Verification items for the finished model (mm, model axes). A direction names the side the tool comes from. Round coordinates to 2 decimals unless told otherwise and drop trailing zeros. Write each loop counter-clockwise with the first axis right and the second up, starting at its lowest first coordinate (ties: lowest second). Pieces come first, ordered by that corner, then holes. Notation, with made-up numbers: M 28,23 L 42,23 A28 ccw 42,57 Z; hole C -16,-30.5 d9. An arc over 180 degrees is marked long. Answer in a Markdown table with one row per item. Add a question column.
1. Sectioned sample at B-B on y = 2.5. Record the cut outline in (x, z).
2. Set-up check for faces 1 (the flat face through (5.45, -1.7, -2.6)), 2 (the flat face through (4.65, -1.7, -2.6)), 3 (the flat face through (5, 14.1, 0)), 4 (the flat face through (2, 11.6, 0.1)), 5 (the flat face through (9.114, 1.674, 2.454)): record each of +Z, -Z, +X, -X, +Y, -Y from which the full face is reachable in a straight line by a thin tool's end or side.
3. Draft check along Y on faces 6 (the flat face through (9.114, 4.826, -2.546)), 7 (the flat face through (5, -2, -2.034)), 8 (the flat face through (5, 13.9, 8)). Enter one of: pulls with the +Y half, pulls with the -Y half, needs draft (parallel to the pull), parting line crosses it, or undercut.
4. Material ranges on probe 1 along Y at (x, z) = (3, -5.75); probe 2 along Y at (x, z) = (5.25, 2); probe 3 along X at (y, z) = (14, 7.44), recorded low to high.
5. Go/stop test with flat-tipped pins: pin 1 Ø5 at (x, z) = (4, -4) entering from -Y; pin 2 Ø1.2 at (x, z) = (5.5, -1.5) entering from +Y; pin 3 Ø1 at (y, z) = (2.5, -2.5) entering from +X. Record where each tip stops, or that it passes through.
6. Sectioned sample at A-A on z = 2.44. Record the cut outline in (x, y).
7. Sectioned sample at D-D on y = 7.25. Record the cut outline in (x, z), plus the area to 3 significant figures.
8. Sectioned sample at C-C on z = -0.25. Record the cut outline in (x, y).
```python
from build123d import *

# Parameters (mm, degrees)
BOSS_EXTRUDE1_DEPTH          = 10.16
FILLET1_R                    = 0.5
CUT_EXTRUDE1_DEPTH           = 21.100885553
CUT_EXTRUDE1_DEPTH_BACK      = 0.2
SKETCH2_R                    = 1.75
SKETCH3_W                    = 0.8
SKETCH3_H                    = 1.05200998
BOSS_EXTRUDE2_DEPTH          = 3.5
SKETCH4_W                    = 2
SKETCH4_H                    = 3.5
CUT_EXTRUDE2_DEPTH           = 2
CUT_EXTRUDE2_DRAFT           = -10
CUT_EXTRUDE2_PROFILE_2_DEPTH = 2
CUT_EXTRUDE2_PROFILE_2_DRAFT = -10
CUT_EXTRUDE2_PROFILE_3_DEPTH = 2
CUT_EXTRUDE2_PROFILE_3_DRAFT = -10
CUT_EXTRUDE2_PROFILE_4_DEPTH = 2
CUT_EXTRUDE2_PROFILE_4_DRAFT = -10
SKETCH5_W                    = 4.000724796
SKETCH5_H                    = 0.5
CUT_EXTRUDE3_DEPTH           = 0.1


with BuildPart() as part:
    # Sketch1 → Boss-Extrude1 (new, symmetric)
    with BuildSketch(Plane.XY):
        Polygon((0, 9.1), (1.5, 9.1), (2.5, 14.1), (8, 14.1), (9.4, 7), (10.1, 7), (10.1, 0), (0, 0), align=None)
    extrude(amount=BOSS_EXTRUDE1_DEPTH, both=True)

    # Fillet1
    fillet1_edges = [part.edges().sort_by_distance(p)[0] for p in [
        (10.1, 7, 0),
    ]]
    fillet(fillet1_edges, radius=FILLET1_R)

    # Sketch2 → Cut-Extrude1 (cut, two sides: drawn at the far end of the back side and taken through both)
    with BuildSketch(Plane(origin=(0, 14.1, 0), x_dir=(1, 0, 0), z_dir=(0, 1, 0)).offset(-CUT_EXTRUDE1_DEPTH_BACK)):
        with Locations(Location((5.25, 7.56, 0), (0, 0, 90))):
            Circle(SKETCH2_R)
        with Locations(Location((5.25, 2.56, 0), (0, 0, 90))):
            Circle(SKETCH2_R)
        with Locations(Location((5.25, -2.44, 0), (0, 0, 90))):
            Circle(SKETCH2_R)
        with Locations(Location((5.25, -7.44, 0), (0, 0, 90))):
            Circle(SKETCH2_R)
    extrude(amount=CUT_EXTRUDE1_DEPTH + CUT_EXTRUDE1_DEPTH_BACK, mode=Mode.SUBTRACT)

    # Sketch3 → Boss-Extrude2 (add)
    with BuildSketch(Plane.XZ):
        with Locations((5.05, 7.44)):
            Rectangle(SKETCH3_W, SKETCH3_H)
        with Locations((5.05, 2.44)):
            Rectangle(SKETCH3_W, SKETCH3_H)
        with Locations((5.05, -2.56)):
            Rectangle(SKETCH3_W, SKETCH3_H)
        with Locations((5.05, -7.56)):
            Rectangle(SKETCH3_W, SKETCH3_H)
    extrude(amount=BOSS_EXTRUDE2_DEPTH)


with BuildPart() as cut_extrude2_tool:
    # Sketch4 → Cut-Extrude2 (with draft: the straight prism first)
    with BuildSketch(Plane(origin=(10.1, 0, 0), x_dir=(0, 0, -1), z_dir=(1, 0, 0))):
        with Locations((-2.44, 3.25)):
            Rectangle(SKETCH4_W, SKETCH4_H)
    extrude(amount=-CUT_EXTRUDE2_DEPTH)
    # Cut-Extrude2: the draft: its side faces are tilted about the plane it starts from
    cut_extrude2_sides = [cut_extrude2_tool.faces().sort_by_distance(p)[0] for p in [
        (9.1, 3.25, 3.44),
        (9.1, 1.5, 2.44),
        (9.1, 3.25, 1.44),
        (9.1, 5, 2.44),
    ]]
    draft(cut_extrude2_sides, Plane(origin=(10.1, 0, 0), x_dir=(0, 0, -1), z_dir=(1, 0, 0)), CUT_EXTRUDE2_DRAFT)


with BuildPart() as part_1:
    add(part.part)

    # Cut-Extrude2: cut by cut_extrude2_tool
    add(cut_extrude2_tool.part, mode=Mode.SUBTRACT)


with BuildPart() as cut_extrude2_profile_2_tool:
    # Sketch4 → Cut-Extrude2 profile 2 (with draft: the straight prism first)
    with BuildSketch(Plane(origin=(10.1, 0, 0), x_dir=(0, 0, -1), z_dir=(1, 0, 0))):
        with Locations((-7.44, 3.25)):
            Rectangle(SKETCH4_W, SKETCH4_H)
    extrude(amount=-CUT_EXTRUDE2_PROFILE_2_DEPTH)
    # Cut-Extrude2 profile 2: the draft: its side faces are tilted about the plane it starts from
    cut_extrude2_profile_2_sides = [cut_extrude2_profile_2_tool.faces().sort_by_distance(p)[0] for p in [
        (9.1, 3.25, 8.44),
        (9.1, 1.5, 7.44),
        (9.1, 3.25, 6.44),
        (9.1, 5, 7.44),
    ]]
    draft(cut_extrude2_profile_2_sides, Plane(origin=(10.1, 0, 0), x_dir=(0, 0, -1), z_dir=(1, 0, 0)), CUT_EXTRUDE2_PROFILE_2_DRAFT)


with BuildPart() as part_2:
    add(part_1.part)

    # Cut-Extrude2 profile 2: cut by cut_extrude2_profile_2_tool
    add(cut_extrude2_profile_2_tool.part, mode=Mode.SUBTRACT)


with BuildPart() as cut_extrude2_profile_3_tool:
    # Sketch4 → Cut-Extrude2 profile 3 (with draft: the straight prism first)
    with BuildSketch(Plane(origin=(10.1, 0, 0), x_dir=(0, 0, -1), z_dir=(1, 0, 0))):
        with Locations((2.56, 3.25)):
            Rectangle(SKETCH4_W, SKETCH4_H)
    extrude(amount=-CUT_EXTRUDE2_PROFILE_3_DEPTH)
    # Cut-Extrude2 profile 3: the draft: its side faces are tilted about the plane it starts from
    cut_extrude2_profile_3_sides = [cut_extrude2_profile_3_tool.faces().sort_by_distance(p)[0] for p in [
        (9.1, 3.25, -1.56),
        (9.1, 1.5, -2.56),
        (9.1, 3.25, -3.56),
        (9.1, 5, -2.56),
    ]]
    draft(cut_extrude2_profile_3_sides, Plane(origin=(10.1, 0, 0), x_dir=(0, 0, -1), z_dir=(1, 0, 0)), CUT_EXTRUDE2_PROFILE_3_DRAFT)


with BuildPart() as part_3:
    add(part_2.part)

    # Cut-Extrude2 profile 3: cut by cut_extrude2_profile_3_tool
    add(cut_extrude2_profile_3_tool.part, mode=Mode.SUBTRACT)


with BuildPart() as cut_extrude2_profile_4_tool:
    # Sketch4 → Cut-Extrude2 profile 4 (with draft: the straight prism first)
    with BuildSketch(Plane(origin=(10.1, 0, 0), x_dir=(0, 0, -1), z_dir=(1, 0, 0))):
        with Locations((7.56, 3.25)):
            Rectangle(SKETCH4_W, SKETCH4_H)
    extrude(amount=-CUT_EXTRUDE2_PROFILE_4_DEPTH)
    # Cut-Extrude2 profile 4: the draft: its side faces are tilted about the plane it starts from
    cut_extrude2_profile_4_sides = [cut_extrude2_profile_4_tool.faces().sort_by_distance(p)[0] for p in [
        (9.1, 3.25, -6.56),
        (9.1, 1.5, -7.56),
        (9.1, 3.25, -8.56),
        (9.1, 5, -7.56),
    ]]
    draft(cut_extrude2_profile_4_sides, Plane(origin=(10.1, 0, 0), x_dir=(0, 0, -1), z_dir=(1, 0, 0)), CUT_EXTRUDE2_PROFILE_4_DRAFT)


with BuildPart() as part_4:
    add(part_3.part)

    # Cut-Extrude2 profile 4: cut by cut_extrude2_profile_4_tool
    add(cut_extrude2_profile_4_tool.part, mode=Mode.SUBTRACT)

    # Sketch5 → Cut-Extrude3 (cut)
    with BuildSketch(Plane(origin=(0, 13.9, 0), x_dir=(1, 0, 0), z_dir=(0, 1, 0))):
        with BuildLine():
            Line((6.982050808, 7.81), (3.517949192, 7.81))
            ThreePointArc((3.517949192, 7.81), (3.5, 7.56), (3.517949192, 7.31))
            Line((3.517949192, 7.31), (6.982050808, 7.31))
            ThreePointArc((6.982050808, 7.31), (6.995506934, 7.434678241), (7, 7.56))
            ThreePointArc((7, 7.56), (6.995506934, 7.685321759), (6.982050808, 7.81))
        make_face()
        with BuildLine():
            Line((6.982050808, -7.19), (3.517949192, -7.19))
            ThreePointArc((3.517949192, -7.19), (3.5, -7.44), (3.517949192, -7.69))
            Line((3.517949192, -7.69), (6.982050808, -7.69))
            ThreePointArc((6.982050808, -7.69), (6.995506934, -7.565321759), (7, -7.44))
            ThreePointArc((7, -7.44), (6.995506934, -7.314678241), (6.982050808, -7.19))
        make_face()
        with Locations((5.343098393, 2.56)):
            Rectangle(SKETCH5_W, SKETCH5_H)
        with Locations((5.343098393, -2.44)):
            Rectangle(SKETCH5_W, SKETCH5_H)
    extrude(amount=-CUT_EXTRUDE3_DEPTH, mode=Mode.SUBTRACT)


solid = part_4.part
```
Geometry check:
| question | item | result |
|---|---|---|
| 1 | outline | M 0,-10.16 L 10.1,-10.16 L 10.1,-8.56 L 8.1,-8.21 L 8.1,-6.91 L 10.1,-6.56 L 10.1,-3.56 L 8.1,-3.21 L 8.1,-1.91 L 10.1,-1.56 L 10.1,1.44 L 8.1,1.79 L 8.1,3.09 L 10.1,3.44 L 10.1,6.44 L 8.1,6.79 L 8.1,8.09 L 10.1,8.44 L 10.1,10.16 L 0,10.16 Z |
| 2 | face 1 | +Z, -Z, +X, -Y |
| 2 | face 2 | +Z, -Z, -X, -Y |
| 2 | face 3 | +Z, -Z, +X, -X, +Y |
| 2 | face 4 | +Z, -Z, -X, +Y |
| 2 | face 5 | +X |
| 3 | face 6 | undercut |
| 3 | face 7 | needs draft |
| 3 | face 8 | pulls with the +Y half |
| 4 | probe 1 | y = 0 to 14.1 |
| 4 | probe 2 | y = -3.5 to 13.9 |
| 4 | probe 3 | x = 2.48 to 3.5, 7 to 8.02 |
| 5 | pin 1 | stops at y = -3.5 |
| 5 | pin 2 | stops at y = 13.9 |
| 5 | pin 3 | stops at x = 8.1 |
| 6 | outline | M 0,0 L 4.65,0 L 4.65,-3.5 L 5.45,-3.5 L 5.45,0 L 10.1,0 L 10.1,1.5 L 8.1,1.85 L 8.1,4.65 L 10.1,5 L 10.1,6.5 A0.5 ccw 9.6,7 L 9.4,7 L 8,14.1 L 7,14.1 L 7,13.9 L 7.34,13.9 L 7.34,13.8 L 3.34,13.8 L 3.34,13.9 L 3.5,13.9 L 3.5,14.1 L 2.5,14.1 L 1.5,9.1 L 0,9.1 Z |
| 7 | outline | M 0,-10.16 L 9.35,-10.16 L 9.35,10.16 L 0,10.16 Z |
| 7 | area | 190 mm2 |
| 8 | outline | M 0,0 L 10.1,0 L 10.1,6.5 A0.5 ccw 9.6,7 L 9.4,7 L 8,14.1 L 2.5,14.1 L 1.5,9.1 L 0,9.1 Z |
